```python
from build123d import *

# Parameters (mm, degrees)
SZKIC1_R                    = 22.5
DODANIE_WYCI_GNI_CIE2_DEPTH = 13
SZKIC2_W                    = 220
SZKIC2_H                    = 30
DODANIE_WYCI_GNI_CIE3_DEPTH = 6
ZAOKR_GLENIE1_R             = 10
SZKIC4_R                    = 20.5
WYTNIJ_WYCI_GNI_CIE3_DEPTH  = 11
WYTNIJ_WYCI_GNI_CIE2_DEPTH  = 4
WYTNIJ_WYCI_GNI_CIE4_REACH  = 173.975
SZKIC8_W                    = 23
SZKIC8_H                    = 13
SZKIC12_R                   = 3.3
DODANIE_WYCI_GNI_CIE4_DEPTH = 3
OTW_R_POD_RUB_M21_D         = 2.6
OTW_R_POD_RUB_M23_D         = 2.6
SZKIC14_R                   = 3.3
DODANIE_WYCI_GNI_CIE5_DEPTH = 5
OTW_R_POD_RUB_M24_D         = 2.6
SZKIC15_W                   = 6
SZKIC15_H                   = 6
SZKIC15_W_2                 = 4
SZKIC15_H_2                 = 4
DODANIE_WYCI_GNI_CIE6_DEPTH = 10
SZYK_LINIOWY1_COUNT         = 2
SZYK_LINIOWY1_PITCH         = 70
OTW_R_POD_RUB_M25_D         = 2.4


with BuildPart() as part:
    # Szkic1 → Dodanie-wyciągnięcie2 (new body)
    with BuildSketch(Plane.XY):
        with Locations(Location((0, 0, 0), (0, 0, 180))):
            Circle(SZKIC1_R)
    extrude(amount=DODANIE_WYCI_GNI_CIE2_DEPTH)

    # Szkic2 → Dodanie-wyciągnięcie3 (add)
    with BuildSketch(Plane.XY):
        with Locations((60, 0)):
            Rectangle(SZKIC2_W, SZKIC2_H)
    extrude(amount=DODANIE_WYCI_GNI_CIE3_DEPTH)

    # Zaokrąglenie1
    zaokr_glenie1_edges = [part.edges().sort_by_distance(p)[0] for p in [
        (170, 15, 3),
        (-50, -15, 3),
        (170, -15, 3),
        (-50, 15, 3),
    ]]
    fillet(zaokr_glenie1_edges, radius=ZAOKR_GLENIE1_R)

    # Szkic4 → Wytnij-wyciągnięcie3 (cut)
    with BuildSketch(Plane.XY.offset(13)):
        Circle(SZKIC4_R)
    extrude(amount=-WYTNIJ_WYCI_GNI_CIE3_DEPTH, mode=Mode.SUBTRACT)

    # Szkic3 → Wytnij-wyciągnięcie2 (cut)
    with BuildSketch(Plane.XY.offset(6)):
        with BuildLine():
            Line((168, -5), (168, 5))
            ThreePointArc((168, 5), (165.656854249, 10.656854249), (160, 13))
            Line((160, 13), (20.766559657, 13))
            ThreePointArc((20.766559657, 13), (24.5, 0), (20.766559657, -13))
            Line((20.766559657, -13), (160, -13))
            ThreePointArc((160, -13), (165.656854249, -10.656854249), (168, -5))
        make_face()
        with BuildLine():
            Line((-48, 5), (-48, -5))
            ThreePointArc((-48, -5), (-45.656854249, -10.656854249), (-40, -13))
            Line((-40, -13), (-20.766559657, -13))
            ThreePointArc((-20.766559657, -13), (-24.5, 0), (-20.766559657, 13))
            Line((-20.766559657, 13), (-40, 13))
            ThreePointArc((-40, 13), (-45.656854249, 10.656854249), (-48, 5))
        make_face()
    extrude(amount=-WYTNIJ_WYCI_GNI_CIE2_DEPTH, mode=Mode.SUBTRACT)

    # Szkic8 → Wytnij-wyciągnięcie4 (cut, up to next)
    with BuildSketch(Plane.XY, mode=Mode.PRIVATE) as wytnij_wyci_gni_cie4_sk1:
        with Locations((150, 0)):
            Rectangle(SZKIC8_W, SZKIC8_H)
    wytnij_wyci_gni_cie4_tool1 = extrude(wytnij_wyci_gni_cie4_sk1.sketch, amount=WYTNIJ_WYCI_GNI_CIE4_REACH, mode=Mode.PRIVATE) & part.part
    add(wytnij_wyci_gni_cie4_tool1.solids().sort_by_distance((150, 0, 0))[0], mode=Mode.SUBTRACT)

    # Szkic12 → Dodanie-wyciągnięcie4 (add)
    with BuildSketch(Plane.XY.offset(2)):
        Circle(SZKIC12_R)
    extrude(amount=DODANIE_WYCI_GNI_CIE4_DEPTH)

    # Otwór pod śrubę M21 (through all)
    with Locations(Plane(origin=(0, 0, 0), x_dir=(1, 0, 0), z_dir=(0, 0, -1))):
        with Locations((0, 0)):
            Hole(OTW_R_POD_RUB_M21_D / 2)

    # Otwór pod śrubę M23 (through all)
    with Locations(Plane(origin=(0, 0, 0), x_dir=(1, 0, 0), z_dir=(0, 0, -1))):
        with Locations((136, 0), (164, 0)):
            Hole(OTW_R_POD_RUB_M23_D / 2)

    # Szkic14 → Dodanie-wyciągnięcie5 (add)
    with BuildSketch(Plane.XY.offset(2)):
        with Locations((-40, 0)):
            Circle(SZKIC14_R)
    extrude(amount=DODANIE_WYCI_GNI_CIE5_DEPTH)

    # Otwór pod śrubę M24 (through all)
    with Locations(Plane(origin=(-40, 0, 0), x_dir=(-1, 0, 0), z_dir=(0, 0, -1))):
        with Locations((0, 0)):
            Hole(OTW_R_POD_RUB_M24_D / 2)

    # Szkic15 → Dodanie-wyciągnięcie6 (add)
    with BuildSketch(Plane(origin=(130, 0, 0), x_dir=(0, 0, -1), z_dir=(1, 0, 0))):
        with Locations((-3, 18)):
            Rectangle(SZKIC15_W, SZKIC15_H)
        with Locations((-3, 18)):
            Rectangle(SZKIC15_W_2, SZKIC15_H_2, mode=Mode.SUBTRACT)
    dodanie_wyci_gni_cie6 = extrude(amount=-DODANIE_WYCI_GNI_CIE6_DEPTH)

    # Szyk liniowy1: Dodanie-wyciągnięcie6 ×2
    with Locations(*[(-i * SZYK_LINIOWY1_PITCH, 0, 0) for i in range(1, SZYK_LINIOWY1_COUNT)]):
        add(dodanie_wyci_gni_cie6)

    # Otwór pod śrubę M25 (through all)
    with Locations(Plane.XY.offset(2)):
        with Locations((55, -10), (105, -10), (105, 10), (55, 10)):
            Hole(OTW_R_POD_RUB_M25_D / 2)

    # Cięcie powierzchnią1
    split(bisect_by=Plane(origin=(80, 0, 0), x_dir=(0, 0, -1), z_dir=(1, 0, 0)), keep=Keep.TOP)


solid = part.part
```
Work out the finished part from the listing and answer in its coordinate system (mm). A direction names the side the tool comes from. Give positions to 0.01 mm unless a question says otherwise; leave off trailing zeros. Loops run counter-clockwise (first coordinate to the right, second up) from the corner with the lowest first, then second, coordinate; pieces in that order, holes last. Notation, with made-up numbers: (-2.5, 89.25) -> (50.5, 89.25) arc R20 cw to (50.5, 119.25) -> close; hole circle Ø7 at (25.25, 62). An arc over 180 degrees is marked (long way). Put each result on its own line as item: value. Start each with the question number.
Item 1: The part is cut by section B-B (y = 0). Give the vertices of the cut face in (x, z).
Item 2: The part is cut by section A-A (x = 105). Give the vertices of the cut face in (y, z).
Item 3: The part is cut by section D-D (z = 3.7). Give the vertices of the cut face in (x, y), then the cut area to 3 significant figures.
Item 4: The part is cut by section C-C (x = 150.5). Give the vertices of the cut face in (y, z), then the cut area to 3 significant figures.
Item 5: Which of the six approach directions +Z, -Z, +X, -X, +Y, -Y give full straight-line access (tool end or side, diameter ignored) to faces 1 (the face through (165.594, -10.719, 4.028)), 2 (the face through (150, -6.5, 1)), 3 (the face through (125, 20, 3))?
Item 6: Each of these flat-tipped pins is pushed along its axis until it touches: P1, Ø2, axis at y = 9, z = 5, coming from the +X side; P2, Ø3, axis at x = 105, y = -10, coming from the +Z side; P3, Ø3, axis at x = 139.5, z = 2.5, coming from the +Y side. Where does it stop, or does it pass through?
Item 7: The mould has two halves that part along Y. Classify faces 4 (the face through (119, -15, 3)), 5 (the face through (145, 15, 3)), 6 (the face through (125, 16, 3)): released by +Y, released by -Y, zero draft, split by the parting line, or undercut.
Item 8: Find the intervals of material crossed by L1, parallel to Y at x = 108, z = 3.2; L2, parallel to Z at x = 125, y = 1; L3, parallel to Y at x = 136, z = 1.55, in increasing order. Write a range as [from, to].
Answers below:
1. outline: (80, 0) -> (134.7, 0) -> (134.7, 2) -> (80, 2) -> close; (137.3, 0) -> (138.5, 0) -> (138.5, 2) -> (137.3, 2) -> close; (161.5, 0) -> (162.7, 0) -> (162.7, 2) -> (161.5, 2) -> close; (165.3, 0) -> (170, 0) -> (170, 6) -> (168, 6) -> (168, 2) -> (165.3, 2) -> close
2. outline: (-15, 0) -> (-11.2, 0) -> (-11.2, 2) -> (-13, 2) -> (-13, 6) -> (-15, 6) -> close; (-8.8, 0) -> (8.8, 0) -> (8.8, 2) -> (-8.8, 2) -> close; (11.2, 0) -> (15, 0) -> (15, 6) -> (13, 6) -> (13, 2) -> (11.2, 2) -> close
3. outline: (80, -15) -> (160, -15) arc R10 ccw to (170, -5) -> (170, 5) arc R10 ccw to (160, 15) -> (130, 15) -> (130, 16) -> (120, 16) -> (120, 15) -> (80, 15) -> (80, 13) -> (160, 13) arc R8 cw to (168, 5) -> (168, -5) arc R8 cw to (160, -13) -> (80, -13) -> close; (120, 20) -> (130, 20) -> (130, 21) -> (120, 21) -> close
3. area: 417 mm2
4. outline: (-15, 0) -> (-6.5, 0) -> (-6.5, 2) -> (-13, 2) -> (-13, 6) -> (-15, 6) -> close; (6.5, 0) -> (15, 0) -> (15, 6) -> (13, 6) -> (13, 2) -> (6.5, 2) -> close
4. area: 50.0 mm2
5. face 1: +Z, -X
5. face 2: +Z, -Z
5. face 3: +X, -X
6. P1: x = 169.54
6. P2: z = 2
6. P3: y = 15
7. face 4: released by -Y
7. face 5: released by +Y
7. face 6: undercut
8. L1: [-15, -13], [13, 15]
8. L2: [0, 2]
8. L3: [-15, -1.3], [1.3, 15]
